Check sheet for the modelled part. Datum: model origin and axes. Units: mm. Coordinates: 2 decimals unless noted, no trailing zeros. Order: outer loops, then holes, each group sorted by start corner. A loop starts at its lowest first (then second) coordinate and runs counter-clockwise, first axis right, second up.
1. Cross-section at B-B (y = -14.25). Enter the section's corners in (x, z) (3 decimals), then the cut area to 3 significant figures.
2. Cross-section at C-C (z = 8). Enter the section's corners in (x, y) (3 decimals).
3. Cross-section at D-D (x = -22.5). Enter the section's corners in (y, z) (3 decimals).
4. Thickness scan on line 1 (Z direction, x = -23.57, y = -8.5) (3 decimals); line 2 (Z direction, x = 0, y = -8) (3 decimals). Record the ranges inside material, lowest first.
5. Cross-section at A-A (x = 0). Enter the section's corners in (y, z) (3 decimals), then the cut area to 3 significant figures.
6. Gauge pin test, flat ends, axial feed: pin 1 Ø1 at (y, z) = (-6.5, 13) entering from -X (3 decimals); pin 2 Ø6.5 at (x, z) = (23.57, -23.57) entering from +Y (3 decimals); pin 3 Ø1.5 at (y, z) = (-2.5, -3.5) entering from -X (3 decimals). Record the tip position at first contact, or that the pin passes through.
7. Draft check along Z on faces 1 (the flat face through (0, -9, 29.845)), 2 (the cylindrical face through (20.95, -11.96, -22.74)), 3 (the flat face through (-29.845, -15, 0)). Enter one of: released by +Z, released by -Z, zero draft, split by the parting line, or undercut.
```python
from build123d import *

# Parameters (mm, degrees)
F0_W     = 59.69
F0_H     = 59.69
F1_DEPTH = 19.05
F2_R     = 19.7430645089
F3_DEPTH = 25.4
F5_D     = 5.5
F8_DEPTH = 59.691


with BuildPart() as f1:
    # F0 (on Front) → F1 (new body)
    with BuildSketch(Plane.XZ):
        Rectangle(F0_W, F0_H)
    extrude(amount=F1_DEPTH)

    # F2 (on face) → F3 (cut)
    with BuildSketch(Plane.XZ.offset(19.05)):
        Circle(F2_R)
    extrude(amount=-F3_DEPTH, mode=Mode.SUBTRACT)

    # F5 (through all)
    with Locations(Plane.XZ.offset(19.05)):
        with Locations((-23.57, 23.57), (23.57, 23.57), (23.57, -23.57), (-23.57, -23.57)):
            Hole(F5_D / 2)

    # F7 (on face) → F8 (cut, through all)
    with BuildSketch(Plane.XY.offset(29.845)):
        Polygon((-29.845, 0), (-29.845, -10.16), (-19.685, 0), align=None)
        Polygon((19.685, 0), (29.845, -10.16), (29.845, 0), align=None)
    extrude(amount=-F8_DEPTH, mode=Mode.SUBTRACT)


solid = f1.part
```
Data:
1. outline: (-29.845, -29.845) - (29.845, -29.845) - (29.845, 29.845) - (-29.845, 29.845) - close; hole circle Ø5.5 at (-23.57, -23.57); hole circle Ø5.5 at (-23.57, 23.57); hole circle Ø39.486 at (0, 0); hole circle Ø5.5 at (23.57, -23.57); hole circle Ø5.5 at (23.57, 23.57)
1. area: 2,240 mm2
2. outline: (-29.845, -19.05) - (-18.05, -19.05) - (-18.05, 0) - (-19.685, 0) - (-29.845, -10.16) - close; (18.05, -19.05) - (29.845, -19.05) - (29.845, -10.16) - (19.685, 0) - (18.05, 0) - close
3. outline: (-19.05, -29.845) - (-2.815, -29.845) - (-2.815, -26.103) - (-19.05, -26.103) - close; (-19.05, -21.037) - (-2.815, -21.037) - (-2.815, 21.037) - (-19.05, 21.037) - close; (-19.05, 26.103) - (-2.815, 26.103) - (-2.815, 29.845) - (-19.05, 29.845) - close
4. line 1: z = -29.845 to -26.32, -20.82 to 20.82, 26.32 to 29.845
4. line 2: z = -29.845 to -19.743, 19.743 to 29.845
5. outline: (-19.05, -29.845) - (0, -29.845) - (0, -19.743) - (-19.05, -19.743) - close; (-19.05, 19.743) - (0, 19.743) - (0, 29.845) - (-19.05, 29.845) - close
5. area: 385 mm2
6. pin 1: stops at x = -26.685
6. pin 2: stops at y = -0.635
6. pin 3: stops at x = -22.935
7. face 1: released by +Z
7. face 2: undercut
7. face 3: zero draft
